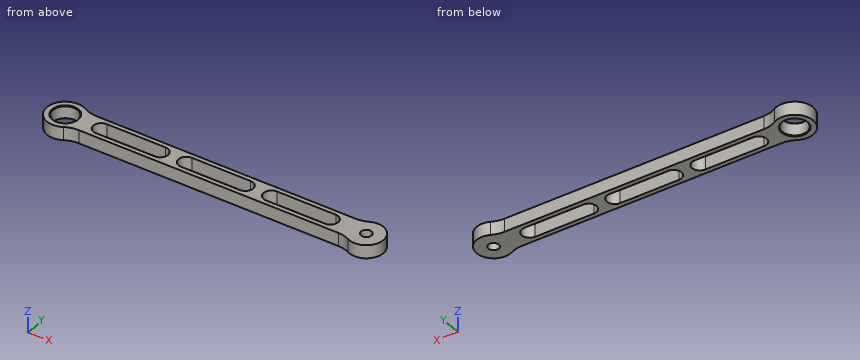
```python
from build123d import *

# Parameters (mm, degrees)
SKETCH_1_R          = 9.5
EXTRUDE_1_DEPTH     = 10
CHAMFER_1_SIZE      = 0.5
CUT_EXTRUDE_2_DEPTH = 10
EXTRUDE_START       = -10
SKETCH_3_R          = 9.5
SKETCH_3_R_2        = 4
EXTRUDE_2_DEPTH     = 10
SKETCH_4_R          = 6
CUT_EXTRUDE_3_DEPTH = 10
SKETCH_5_R          = 6
SKETCH_5_R_2        = 4
EXTRUDE_3_DEPTH     = 10


with BuildPart() as part:
    # 草图1 → 凸台-拉伸1 (new body)
    with BuildSketch(Plane.XY):
        with BuildLine():
            Line((16.904141504, -9.5), (212.802616478, -9.5))
            Line((212.802616478, -9.5), (215.209800542, -9.5))
            ThreePointArc((215.209800542, -9.5), (219.815462407, -10.037526396), (224.173557789, -11.621212121))
            ThreePointArc((224.173557789, -11.621212121), (243, 0), (224.173557789, 11.621212121))
            ThreePointArc((224.173557789, 11.621212121), (219.815462407, 10.037526396), (215.209800542, 9.5))
            Line((215.209800542, 9.5), (212.802616478, 9.5))
            Line((212.802616478, 9.5), (16.904141504, 9.5))
            ThreePointArc((16.904141504, 9.5), (11.75918395, 10.173090993), (6.960528855, 12.147058824))
            ThreePointArc((6.960528855, 12.147058824), (-14, 0), (6.960528855, -12.147058824))
            ThreePointArc((6.960528855, -12.147058824), (11.75918395, -10.173090993), (16.904141504, -9.5))
        make_face()
        Circle(SKETCH_1_R, mode=Mode.SUBTRACT)
        with Locations((230, 0)):
            Circle(SKETCH_1_R, mode=Mode.SUBTRACT)
    extrude(amount=EXTRUDE_1_DEPTH)

    # 倒角1
    chamfer_1_edges = [part.edges().sort_by_distance(p)[0] for p in [
        (-9.5, 0, 0),
        (-9.5, 0, 10),
    ]]
    chamfer(chamfer_1_edges, length=CHAMFER_1_SIZE)

    # 草图2 → 切除-拉伸2 (cut)
    with BuildSketch(Plane.XY.offset(10)):
        with BuildLine():
            Line((137.499999918, -6), (92.5, -6))
            ThreePointArc((92.5, -6), (86.5, 0), (92.5, 6))
            Line((92.5, 6), (137.499999918, 6))
            ThreePointArc((137.499999918, 6), (143.499999918, 0), (137.499999918, -6))
        make_face()
        with BuildLine():
            Line((27.5, -6), (72.5, -6))
            ThreePointArc((72.5, -6), (78.5, 0), (72.5, 6))
            Line((72.5, 6), (27.5, 6))
            ThreePointArc((27.5, 6), (21.5, 0), (27.5, -6))
        make_face()
        with BuildLine():
            Line((157.5, -6), (202.5, -6))
            ThreePointArc((202.5, -6), (208.5, 0), (202.5, 6))
            Line((202.5, 6), (157.5, 6))
            ThreePointArc((157.5, 6), (151.5, 0), (157.5, -6))
        make_face()
    extrude(amount=-CUT_EXTRUDE_2_DEPTH, mode=Mode.SUBTRACT)

    # 草图3 → 凸台-拉伸2 (add)
    with BuildSketch(Plane.XY.offset(10).offset(EXTRUDE_START)):
        with Locations((230, 0)):
            Circle(SKETCH_3_R)
        with Locations((230, 0)):
            Circle(SKETCH_3_R_2, mode=Mode.SUBTRACT)
    extrude(amount=EXTRUDE_2_DEPTH)

    # 草图4 → 切除-拉伸3 (cut)
    with BuildSketch(Plane.XY.offset(10)):
        with Locations((230, 0)):
            Circle(SKETCH_4_R)
    extrude(amount=-CUT_EXTRUDE_3_DEPTH, mode=Mode.SUBTRACT)

    # 草图5 → 凸台-拉伸3 (add)
    with BuildSketch(Plane.XY.offset(10)):
        with Locations((230, 0)):
            Circle(SKETCH_5_R)
        with Locations((230, 0)):
            Circle(SKETCH_5_R_2, mode=Mode.SUBTRACT)
    extrude(amount=-EXTRUDE_3_DEPTH)


solid = part.part
```
Work out the finished part from the listing and answer in its coordinate system (mm). Round coordinates to 2 decimals unless told otherwise and drop trailing zeros. Write each loop counter-clockwise with the first axis right and the second up, starting at its lowest first coordinate (ties: lowest second). Pieces come first, ordered by that corner, then holes.
1) Flat-ended cylindrical pins translate along their axes: P1, Ø6, axis at y = 3.5, z = 3, coming from the +X side; P2, Ø3, axis at x = 91, z = 4.5, coming from the -Y side; P3, Ø4, axis at x = 28, y = -2.5, coming from the -Z side; P4, Ø5, axis at x = 51, z = 3.5, coming from the +Y side. Find the tip coordinate at first contact, or state that the pin passes through.
2) A cutting plane is placed at C-C on z = 4.5. Determine the outline of the cut face in (x, y), and give its area (3 significant figures).
3) Consider probe 1 along Y at (x, z) = (126, 7); probe 2 along Y at (x, z) = (0, 4.25); probe 3 along X at (y, z) = (1.25, 8). Determine where each line is inside the solid, lowest interval first.
4) A cutting plane is placed at A-A on x = 230. Determine the outline of the cut face in (y, z), and give its area (3 significant figures).
5) A cutting plane is placed at D-D on x = 43.5. Determine the outline of the cut face in (y, z), and give its area (3 significant figures).
6) A cutting plane is placed at B-B on y = 0. Determine the outline of the cut face in (x, z), and give its area (4 significant figures).
Entries:
1. P1: stops at x = 242.99
1. P2: stops at y = -9.5
1. P3: passes through
1. P4: stops at y = 9.5
2. outline: (6.96, -12.15) arc R20 cw to (16.9, -9.5) - (215.21, -9.5) arc R20 cw to (224.17, -11.62) arc R13 ccw (long way) to (224.17, 11.62) arc R20 cw to (215.21, 9.5) - (16.9, 9.5) arc R20 cw to (6.96, 12.15) arc R14 ccw (long way) to start; hole circle Ø19 at (0, 0); hole (27.5, -6) - (72.5, -6) arc R6 ccw to (72.5, 6) - (27.5, 6) arc R6 ccw to start; hole (92.5, -6) - (137.5, -6) arc R6 ccw to (137.5, 6) - (92.5, 6) arc R6 ccw to start; hole (157.5, -6) - (202.5, -6) arc R6 ccw to (202.5, 6) - (157.5, 6) arc R6 ccw to start; hole circle Ø8 at (230, 0)
2. area: 2,770 mm2
3. probe 1: y = -9.5 to -6, 6 to 9.5
3. probe 2: y = -14 to -9.5, 9.5 to 14
3. probe 3: x = -13.94 to -9.42, 9.42 to 21.63, 78.37 to 86.63, 143.37 to 151.63, 208.37 to 226.2, 233.8 to 242.94
4. outline: (-13, 0) - (-4, 0) - (-4, 10) - (-13, 10) - close; (4, 0) - (13, 0) - (13, 10) - (4, 10) - close
4. area: 180 mm2
5. outline: (-9.5, 0) - (-6, 0) - (-6, 10) - (-9.5, 10) - close; (6, 0) - (9.5, 0) - (9.5, 10) - (6, 10) - close
5. area: 70.0 mm2
6. outline: (-14, 0) - (-10, 0) - (-9.5, 0.5) - (-9.5, 9.5) - (-10, 10) - (-14, 10) - close; (9.5, 0.5) - (10, 0) - (21.5, 0) - (21.5, 10) - (10, 10) - (9.5, 9.5) - close; (78.5, 0) - (86.5, 0) - (86.5, 10) - (78.5, 10) - close; (143.5, 0) - (151.5, 0) - (151.5, 10) - (143.5, 10) - close; (208.5, 0) - (226, 0) - (226, 10) - (208.5, 10) - close; (234, 0) - (243, 0) - (243, 10) - (234, 10) - close
6. area: 589.5 mm2
